from build123d import *

# Parameters (mm, degrees)
SKETCH1_W               = 139.7
SKETCH1_H               = 76.2
BOSS_EXTRUDE1_DEPTH     = 38.1
CUT_EXTRUDE1_DEPTH      = 89.217019333
CUT_EXTRUDE1_DEPTH_BACK = 31.75
SKETCH3_R               = 2.032
CUT_EXTRUDE2_DEPTH      = 89.217019333
SKETCH4_W               = 52.07
SKETCH4_H               = 25.4
CUT_EXTRUDE3_DEPTH      = 10.414
SKETCH7_W               = 57.15
SKETCH7_H               = 12.7
BOSS_EXTRUDE2_DEPTH     = 25.4
SKETCH8_W               = 57.15
SKETCH8_H               = 50.8
BOSS_EXTRUDE3_DEPTH     = 12.7
SKETCH5_R               = 2.286
SKETCH5_R_2             = 2.54
CUT_EXTRUDE4_DEPTH      = 109.570070904
CUT_EXTRUDE5_DEPTH      = 14.986
CUT_EXTRUDE6_DEPTH      = 7.112
SKETCH10_R              = 2.159
CUT_EXTRUDE7_DEPTH      = 139.84509874
SKETCH11_W              = 52.07
SKETCH11_H              = 6.35
BOSS_EXTRUDE4_DEPTH     = 25.4
BOSS_EXTRUDE5_DEPTH     = 38.1
SKETCH15_R              = 3.175
CUT_EXTRUDE8_DEPTH      = 6.35
SKETCH16_R              = 3.175
BOSS_EXTRUDE6_DEPTH     = 6.35


with BuildPart() as part:
    # Sketch1 → Boss-Extrude1 (new body)
    with BuildSketch(Plane(origin=(0, 0, 0), x_dir=(1, 0, 0), z_dir=(0, 1, 0))):
        Rectangle(SKETCH1_W, SKETCH1_H)
    extrude(amount=-BOSS_EXTRUDE1_DEPTH)

    # Sketch2 → Cut-Extrude1 (cut, two sides: drawn at the far end of the back side and taken through both)
    with BuildSketch(Plane.XZ.offset(38.1).offset(-CUT_EXTRUDE1_DEPTH_BACK)):
        Polygon((386.759367729, 25.4), (69.85, 25.4), (7.62, 25.4), (7.62, 0), (-58.42, 0), (-58.42, -38.1), (-58.42, -355.009367729), (353.331408797, -836.86719611), (798.510776526, -456.457828381), align=None)
    extrude(amount=CUT_EXTRUDE1_DEPTH + CUT_EXTRUDE1_DEPTH_BACK, mode=Mode.SUBTRACT)

    # Sketch3 → Cut-Extrude2 (cut, through all)
    with BuildSketch(Plane.XZ.offset(38.1)):
        with Locations(Location((-53.34, 21.59, 0), (0, 0, 270))):
            Circle(SKETCH3_R)
    extrude(amount=-CUT_EXTRUDE2_DEPTH, mode=Mode.SUBTRACT)

    # Sketch4 → Cut-Extrude3 (cut)
    with BuildSketch(Plane(origin=(0, 0, 0), x_dir=(-1, 0, 0), z_dir=(0, 0, -1))):
        with Locations((32.385, -19.05)):
            Rectangle(SKETCH4_W, SKETCH4_H)
    extrude(amount=-CUT_EXTRUDE3_DEPTH, mode=Mode.SUBTRACT)

    # Sketch7 → Boss-Extrude2 (add)
    with BuildSketch(Plane.XY.offset(38.1)):
        with Locations((-41.275, -6.35)):
            Rectangle(SKETCH7_W, SKETCH7_H)
    extrude(amount=BOSS_EXTRUDE2_DEPTH)

    # Sketch8 → Boss-Extrude3 (add)
    with BuildSketch(Plane.XY.offset(63.5)):
        with Locations((-41.275, -25.4)):
            Rectangle(SKETCH8_W, SKETCH8_H)
    extrude(amount=BOSS_EXTRUDE3_DEPTH)

    # Sketch5 → Cut-Extrude4 (cut, through all)
    with BuildSketch(Plane(origin=(0, 0, 10.414), x_dir=(-1, 0, 0), z_dir=(0, 0, -1))):
        with Locations((46.99, -19.05)):
            Circle(SKETCH5_R)
        with Locations((34.29, -19.05)):
            Circle(SKETCH5_R_2)
        with Locations((21.59, -19.05)):
            Circle(SKETCH5_R_2)
    extrude(amount=-CUT_EXTRUDE4_DEPTH, mode=Mode.SUBTRACT)

    # Sketch6 → Cut-Extrude5 (cut)
    with BuildSketch(Plane(origin=(0, 0, 10.414), x_dir=(-1, 0, 0), z_dir=(0, 0, -1))):
        with BuildLine():
            Line((27.051, -18.288), (26.612524863, -18.288))
            ThreePointArc((26.612524863, -18.288), (16.51, -19.05), (26.612524863, -19.812))
            Line((26.612524863, -19.812), (27.051, -19.812))
            Line((27.051, -19.812), (27.051, -21.082))
            Line((27.051, -21.082), (28.829, -21.082))
            Line((28.829, -21.082), (28.829, -19.812))
            Line((28.829, -19.812), (29.267475137, -19.812))
            ThreePointArc((29.267475137, -19.812), (39.37, -19.05), (29.267475137, -18.288))
            Line((29.267475137, -18.288), (28.829, -18.288))
            Line((28.829, -18.288), (28.829, -17.018))
            Line((28.829, -17.018), (27.051, -17.018))
            Line((27.051, -17.018), (27.051, -18.288))
        make_face()
    extrude(amount=-CUT_EXTRUDE5_DEPTH, mode=Mode.SUBTRACT)

    # Sketch9 → Cut-Extrude6 (cut)
    with BuildSketch(Plane(origin=(0, 0, 63.5), x_dir=(-1, 0, 0), z_dir=(0, 0, -1))):
        Polygon((42.323188216, -16.865376771), (42.323188216, -46.634623229), (44.704, -49.276), (49.276, -49.276), (51.656811784, -46.634623229), (51.656811784, -16.865376771), (49.276, -14.224), (44.704, -14.224), align=None)
    extrude(amount=-CUT_EXTRUDE6_DEPTH, mode=Mode.SUBTRACT)

    # Sketch10 → Cut-Extrude7 (cut, through all)
    with BuildSketch(Plane(origin=(0, 0, 70.612), x_dir=(-1, 0, 0), z_dir=(0, 0, -1))):
        with Locations((46.99, -19.05)):
            Circle(SKETCH10_R)
        with Locations((46.99, -31.75)):
            Circle(SKETCH10_R)
        with Locations((46.99, -44.45)):
            Circle(SKETCH10_R)
    extrude(amount=-CUT_EXTRUDE7_DEPTH, mode=Mode.SUBTRACT)

    # Sketch11 → Boss-Extrude4 (add)
    with BuildSketch(Plane(origin=(0, 0, 0), x_dir=(-1, 0, 0), z_dir=(0, 0, -1))):
        with Locations((32.385, -34.925)):
            Rectangle(SKETCH11_W, SKETCH11_H)
    extrude(amount=BOSS_EXTRUDE4_DEPTH)

    # Sketch14 → Boss-Extrude5 (add)
    with BuildSketch(Plane(origin=(0, 0, 0), x_dir=(1, 0, 0), z_dir=(0, 1, 0))):
        Polygon((-12.7, -76.2), (25.4, -38.1), (-12.7, -38.1), align=None)
    extrude(amount=-BOSS_EXTRUDE5_DEPTH)

    # Sketch15 → Cut-Extrude8 (cut)
    with BuildSketch(Plane.XZ.offset(38.1)):
        with Locations(Location((57.15, 31.75, 0), (0, 0, 270))):
            Circle(SKETCH15_R)
        with Locations(Location((0.000881951, 32.0675, 0), (0, 0, 270))):
            Circle(SKETCH15_R)
        with Locations(Location((-57.148236098, 32.385, 0), (0, 0, 270))):
            Circle(SKETCH15_R)
    extrude(amount=-CUT_EXTRUDE8_DEPTH, mode=Mode.SUBTRACT)

    # Sketch16 → Boss-Extrude6 (add)
    with BuildSketch(Plane(origin=(0, 0, 0), x_dir=(1, 0, 0), z_dir=(0, 1, 0))):
        with Locations(Location((57.15, -32.258, 0), (0, 0, 90))):
            Circle(SKETCH16_R)
        with Locations(Location((0, -32.258, 0), (0, 0, 90))):
            Circle(SKETCH16_R)
        with Locations(Location((-57.15, -32.258, 0), (0, 0, 90))):
            Circle(SKETCH16_R)
        with Locations(Location((-63.5, 25.4, 0), (0, 0, 90))):
            Circle(SKETCH16_R)
    extrude(amount=BOSS_EXTRUDE6_DEPTH)


solid = part.part
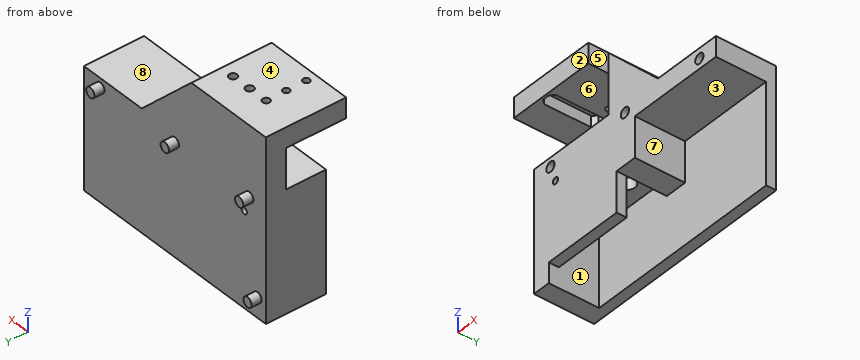
Can you work these out from the model? Positions are in its coordinate system, mm. Face numbers are marked on the shaded views. A direction names the side the tool comes from. Coordinates: 2 decimals unless noted, no trailing zeros. Order: outer loops, then holes, each group sorted by start corner. A loop starts at its lowest first (then second) coordinate and runs counter-clockwise, first axis right, second up. Notation, with made-up numbers: (53.25, 67) - (82.25, 67) arc R6 ccw to (82.25, 71) - close; hole circle Ø11 at (-20, 53). An arc over 180 degrees is marked (long way). Answer as a JSON object with one key per item and string values. Group by question number.
Q1. Imagine slicing it at C-C (y = -9). Please give me the cut outline in (x, z), and give its area (3 significant figures).
Q2. On a 3-axis mill with a long thin cutter (end or side, diameter ignored), from which of +Z, -Z, +X, -X, +Y, -Y can I reach the whole of each face in a straight line? I mean the marked faces 4, 5, 6, 7 and 8. Say none if no direction works.
Q3. I need wall thicknesses on line 1 (Z direction, x = -53, y = -23); line 2 (Y direction, x = -27, z = -3); line 3 (Z direction, x = -13.5, y = -15). Which ranges of each line are inside material? Lowest first, please. Write a range as from..to.
Q4. Imagine slicing it at D-D (z = 7). Please give me the cut outline in (x, y), and give its area (3 significant figures).
Q5. Will these pins go through, and if not, where does the flat tip stop? P1, Ø1, axis at x = -49, z = -16.5, coming from the -Y side; P2, Ø0.5, axis at x = -28, z = 20, coming from the +Y side; P3, Ø6, axis at x = -34.29, y = -19.05, coming from the -Z side; P4, Ø6, axis at x = -12.5, y = -23, coming from the +Z side.
Q6. Imagine slicing it at B-B (x = -46.99). Give the number of separate pieces and of enclosed holes in the cut face, and give its area (3 significant figures).
Q7. We'd pull the mould along Y, two halves only. Please class the marked faces 1, 2 and 3: +Y half, -Y half, draft (parallel to the pull), parting line (faces both ways), or undercut.
Q8. Imagine slicing it at A-A (z = 21.59). Please give me the cut outline in (x, y), and give its area (3 significant figures).
Determined:
{
 "1": {"outline": "(-69.85, -38.1) - (-58.42, -38.1) - (-58.42, 10.41) - (-6.35, 10.41) - (-6.35, 0) - (7.62, 0) - (7.62, 25.4) - (69.85, 25.4) - (69.85, 38.1) - (25.4, 38.1) - (-12.7, 76.2) - (-69.85, 76.2) - close; hole circle Ø4.06 at (-53.34, 21.59)", "area": "6,530 mm2"},
 "2": {"face 4": "+Z, +X, -X, +Y, -Y", "face 5": "+Z, -Z, +X, -Y", "face 6": "-X, -Y", "face 7": "-Z, +X, -Y", "face 8": "+Z, +X, +Y, -Y"},
 "3": {"line 1": "z = 10.41..19.59, 23.59..38.1, 63.5..76.2", "line 2": "y = -38.1..-31.75, -6.35..0", "line 3": "z = 10.41..38.1, 63.5..76.2"},
 "4": {"outline": "(-69.85, -38.1) - (7.62, -38.1) - (7.62, -6.35) - (69.85, -6.35) - (69.85, 0) - (-69.85, 0) - close; hole (-58.42, -31.75) - (-6.35, -31.75) - (-6.35, -6.35) - (-58.42, -6.35) - close", "area": "2,020 mm2"},
 "5": {"P1": "stops at y = -38.1", "P2": "stops at y = 0", "P3": "stops at z = 25.4", "P4": "stops at z = 76.2"},
 "6": {"separate pieces": "5", "enclosed holes": "0", "area": "2,110 mm2"},
 "7": {"face 1": "undercut", "face 2": "-Y half", "face 3": "draft"},
 "8": {"outline": "(-69.85, -38.1) - (-55.37, -38.1) - (-55.37, 0) - (-69.85, 0) - close; (-51.31, -38.1) - (7.62, -38.1) - (7.62, -6.35) - (69.85, -6.35) - (69.85, 0) - (-51.31, 0) - close; hole circle Ø4.57 at (-46.99, -19.05); hole (-29.27, -19.81) - (-28.83, -19.81) - (-28.83, -21.08) - (-27.05, -21.08) - (-27.05, -19.81) - (-26.61, -19.81) arc R5.08 ccw (long way) to (-26.61, -18.29) - (-27.05, -18.29) - (-27.05, -17.02) - (-28.83, -17.02) - (-28.83, -18.29) - (-29.27, -18.29) arc R5.08 ccw (long way) to start", "area": "3,000 mm2"}
}
